Work out the finished part from the listing and answer in its coordinate system (mm). Face numbers are marked on the shaded views. A direction names the side the tool comes from. Round coordinates to 2 decimals unless told otherwise and drop trailing zeros. Order: outer loops, then holes, each group sorted by start corner. A loop starts at its lowest first (then second) coordinate and runs counter-clockwise, first axis right, second up.
from build123d import *

# Parameters (mm, degrees)
PAD042_DEPTH             = 3
CLONE021_PLACEMENT_ANGLE = 90
CYLINDER1056_R           = 1
CYLINDER1056_DEPTH       = 5
CYLINDER1057_R           = 1
CYLINDER1057_DEPTH       = 5
BOX265_W                 = 27
BOX265_H                 = 16
BOX265_DEPTH             = 1.5


with BuildPart() as obj1:
    # Sketch067 → Pad042 (new body, symmetric)
    with BuildSketch(Plane(origin=(13, 8, 1.5), x_dir=(0, 0, 1), z_dir=(0, -1, 0))):
        Polygon((0, 0), (10, 0), (10, 3.8), (1.85, 3.8), (1.85, 8.8), (10, 8.8), (10, 12.6), (0, 12.6), align=None)
    extrude(amount=PAD042_DEPTH, both=True)


with BuildPart() as obj1_1:
    # Clone021 placement: moved
    add(obj1.part.moved(Location((11, 1.3, 0))).rotate(Axis((11, 1.3, 0), (0, 0, 1)), CLONE021_PLACEMENT_ANGLE))


with BuildPart() as cylinder1094:
    # Cylinder1056 → Cylinder1056 (new body)
    with BuildSketch(Plane(origin=(24, 3, 0), x_dir=(1, 0, 0), z_dir=(0, 0, 1))):
        Circle(CYLINDER1056_R)
    extrude(amount=CYLINDER1056_DEPTH)


with BuildPart() as fusion153:
    # Cylinder1057 → Cylinder1057 (new body)
    with BuildSketch(Plane(origin=(24, 13, 0), x_dir=(1, 0, 0), z_dir=(0, 0, 1))):
        Circle(CYLINDER1057_R)
    extrude(amount=CYLINDER1057_DEPTH)

    # Fusion153: union Cylinder1094
    add(cylinder1094.part)


with BuildPart() as obj2:
    # Box265 → Box265 (new body)
    with BuildSketch(Plane.XY):
        with Locations((13.5, 8)):
            Rectangle(BOX265_W, BOX265_H)
    extrude(amount=BOX265_DEPTH)

    # Cut137: cut Fusion153
    add(fusion153.part, mode=Mode.SUBTRACT)

    # Fusion: union obj1
    add(obj1_1.part)


solid = obj2.part
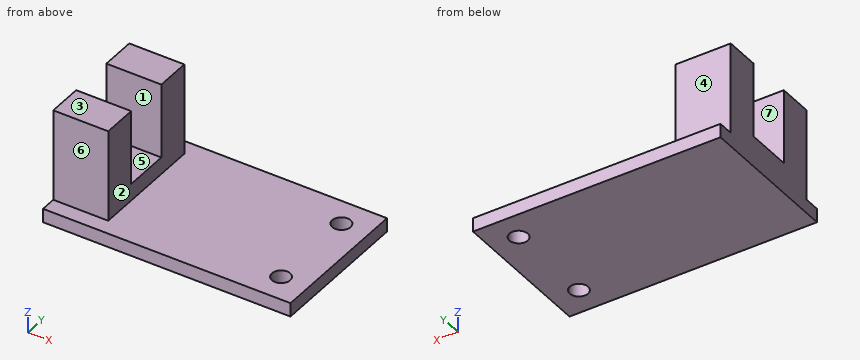
Item 1: Find section C-C (y = 3). Write down the section's boundary in (x, z), plus the area to 3 significant figures.
Item 2: Find section A-A (z = 7.5). Write down the section's boundary in (x, y).
Item 3: Given pin 1 (1.8 mm diameter, centred on x = 24, y = 3, fed in from +Z); pin 2 (1.8 mm diameter, centred on x = 3.5, z = 8, fed in from -Y); pin 3 (5 mm diameter, centred on x = 3, z = 7, fed in from +Y); pin 4 (1.5 mm diameter, centred on x = 2, y = 7, fed in from +Z), each flat-ended and moving along its own axis, determine where each tip first touches the part or whether it passes through.
Item 4: For a pull along Y with two mould halves and no side action, classify the marked faces 4, 5, 6 and 7 as released by +Y, released by -Y, zero draft, split by the parting line, or undercut.
Item 5: Find the intervals of material crossed by line 1 along Y through (x, z) = (24, 0.5); line 2 along X through (y, z) = (3, 0.9); line 3 along Z through (x, y) = (9, 2.75), in increasing order.
Item 6: Find section B-B (x = 24). Write down the section's boundary in (y, z), plus the area to 3 significant figures.
Item 7: Find section D-D (x = 4.5). Write down the section's boundary in (y, z).
Item 8: A tool of negligible diameter and unlimited length cuts with its end or side. For the marked faces 1, 2 and 3, from which of +Z, -Z, +X, -X, +Y, -Y can it reach the whole face along a straight path? Write none if from no direction.
Model answer:
1. outline: (0, 0) - (23, 0) - (23, 1.5) - (6, 1.5) - (6, 11.5) - (0, 11.5) - close; (25, 0) - (27, 0) - (27, 1.5) - (25, 1.5) - close
1. area: 97.5 mm2
2. outline: (0, 1.7) - (6, 1.7) - (6, 5.5) - (0, 5.5) - close; (0, 10.5) - (6, 10.5) - (6, 14.3) - (0, 14.3) - close
3. pin 1: passes through
3. pin 2: stops at y = 1.7
3. pin 3: stops at y = 14.3
3. pin 4: stops at z = 3.35
4. face 4: released by +Y
4. face 5: undercut
4. face 6: released by -Y
4. face 7: undercut
5. line 1: y = 0 to 2, 4 to 12, 14 to 16
5. line 2: x = 0 to 23, 25 to 27
5. line 3: z = 0 to 1.5
6. outline: (0, 0) - (2, 0) - (2, 1.5) - (0, 1.5) - close; (4, 0) - (12, 0) - (12, 1.5) - (4, 1.5) - close; (14, 0) - (16, 0) - (16, 1.5) - (14, 1.5) - close
6. area: 18.0 mm2
7. outline: (0, 0) - (16, 0) - (16, 1.5) - (14.3, 1.5) - (14.3, 11.5) - (10.5, 11.5) - (10.5, 3.35) - (5.5, 3.35) - (5.5, 11.5) - (1.7, 11.5) - (1.7, 1.5) - (0, 1.5) - close
8. face 1: +Z, +X, -X
8. face 2: +Z, +X, +Y, -Y
8. face 3: +Z, +X, -X, +Y, -Y
